Could you check a few things on this model? Use its own coordinates, in mm. Coordinates: 2 decimals unless noted, no trailing zeros. Write each loop counter-clockwise with the first axis right and the second up, starting at its lowest first coordinate (ties: lowest second). Pieces come first, ordered by that corner, then holes. Notation, with made-up numbers: M 17.25,73 L 24.25,73 A13 ccw 24.25,83 Z; hole C -16.5,38.5 d2. An arc over 180 degrees is marked long. Write item = value, one per line.
```python
from build123d import *

# Parameters (mm, degrees)
SKETCH_1_R      = 1.5
EXTRUDE_1_DEPTH = 30


with BuildPart() as part:
    # 草图1 → 凸台-拉伸1 (new body)
    with BuildSketch(Plane(origin=(0, 0, 0), x_dir=(1, 0, 0), z_dir=(0, 1, 0))):
        with BuildLine():
            Line((0, 0), (-5.900613322, -17.701839967))
            ThreePointArc((-5.900613322, -17.701839967), (-10.674994221, -19.051316702), (-7.665175543, -22.995526629))
            Line((-7.665175543, -22.995526629), (-17.567279989, -52.701839967))
            ThreePointArc((-17.567279989, -52.701839967), (-22.341660888, -54.051316702), (-19.33184221, -57.995526629))
            Line((-19.33184221, -57.995526629), (-20, -60))
            Line((-20, -60), (-18, -60))
            Line((-18, -60), (2, 0))
            Line((2, 0), (2, 20))
            Line((2, 20), (0, 20))
            Line((0, 20), (0, 17.828427125))
            ThreePointArc((0, 17.828427125), (-4, 15), (0, 12.171572875))
            Line((0, 12.171572875), (0, 0))
        make_face()
        with Locations(Location((-7.828944327, -20, 0), (0, 0, 270))):
            Circle(SKETCH_1_R, mode=Mode.SUBTRACT)
        with Locations(Location((-1, 15, 0), (0, 0, 270))):
            Circle(SKETCH_1_R, mode=Mode.SUBTRACT)
        with Locations(Location((-19.495610994, -55, 0), (0, 0, 270))):
            Circle(SKETCH_1_R, mode=Mode.SUBTRACT)
    extrude(amount=EXTRUDE_1_DEPTH)


solid = part.part
```
Item 1: Imagine slicing it at D-D (z = -4.5). Write out the boundary of the cut face in (x, y).
Numbers:
outline = M 0,0 L 2,0 L 2,30 L 0,30 Z
Item 2: If I drill on line 1 along X through (y, z) = (14.75, -15); line 2 along X through (y, z) = (7, -10); line 3 along Z through (x, y) = (-20.25, 22.25), over which ranges is the centre line in solid material (lowest first)?
Numbers:
line_1 = -4 to -2.5, 0.5 to 2
line_2 = 0 to 2
line_3 = 52.1 to 53.7, 56.3 to 57.9
Item 3: I'm going to push flat-ended pins straight in: P1, Ø10, axis at x = -7, z = 39.5, coming from the +Y side; P2, Ø8, axis at y = 9.5, z = 25, coming from the -X side; P3, Ø12, axis at x = -10, z = 6.5, coming from the +Y side; P4, Ø3.5, axis at y = 16.5, z = -7.5, coming from the -X side. Where does each tip first touch, or does it pass through?
Numbers:
P1 = 30
P2 = -10.66
P3 = through
P4 = 0
Item 4: Imagine slicing it at C-C (y = 12.5). Write out the boundary of the cut face in (x, z), and give its area (3 significant figures).
Numbers:
outline = M -20,60 L -19.33,58 A3 ccw long -17.57,52.7 L -7.67,23 A3 ccw long -5.9,17.7 L 0,0 L 0,-12.17 A3 ccw long 0,-17.83 L 0,-20 L 2,-20 L 2,0 L -18,60 Z; hole C -19.5,55 d3; hole C -7.83,20 d3; hole C -1,-15 d3
area = 200 mm²
Item 5: Imagine slicing it at A-A (x = -1). Write out the boundary of the cut face in (y, z), and give its area (3 significant figures).
Numbers:
outline = M 0,-18 L 30,-18 L 30,-16.5 L 0,-16.5 Z; M 0,-13.5 L 30,-13.5 L 30,-12 L 0,-12 Z; M 0,3 L 30,3 L 30,9 L 0,9 Z
area = 270 mm²
Item 6: Imagine slicing it at B-B (z = -15). Write out the boundary of the cut face in (x, y), and give its area (3 significant figures).
Numbers:
outline = M -4,0 L -2.5,0 L -2.5,30 L -4,30 Z; M 0.5,0 L 2,0 L 2,30 L 0.5,30 Z
area = 90.0 mm²
Item 7: If we mould it in two halves opening along Z, with no side actions, what happens to faces 1 (the face through (-10.648, 14.79, 18.974)), 2 (the face through (-20.07, 14.79, 56.386)), 3 (the face through (-7.6, 30, 22.8)), 4 (the face through (-19, 15, 60))? For each: pulls with the +Z half, pulls with the -Z half, needs draft (parallel to the pull), parting line crosses it, or undercut.
Numbers:
face_1 = undercut
face_2 = undercut
face_3 = needs draft
face_4 = pulls with the +Z half
